Can you work these out from the drawing? Everything is in mm from the part's minimum corner. Coordinates: 2 decimals unless noted, no trailing zeros. Write each loop counter-clockwise with the first axis right and the second up, starting at its lowest first coordinate (ties: lowest second). Pieces come first, ordered by that corner, then holes.
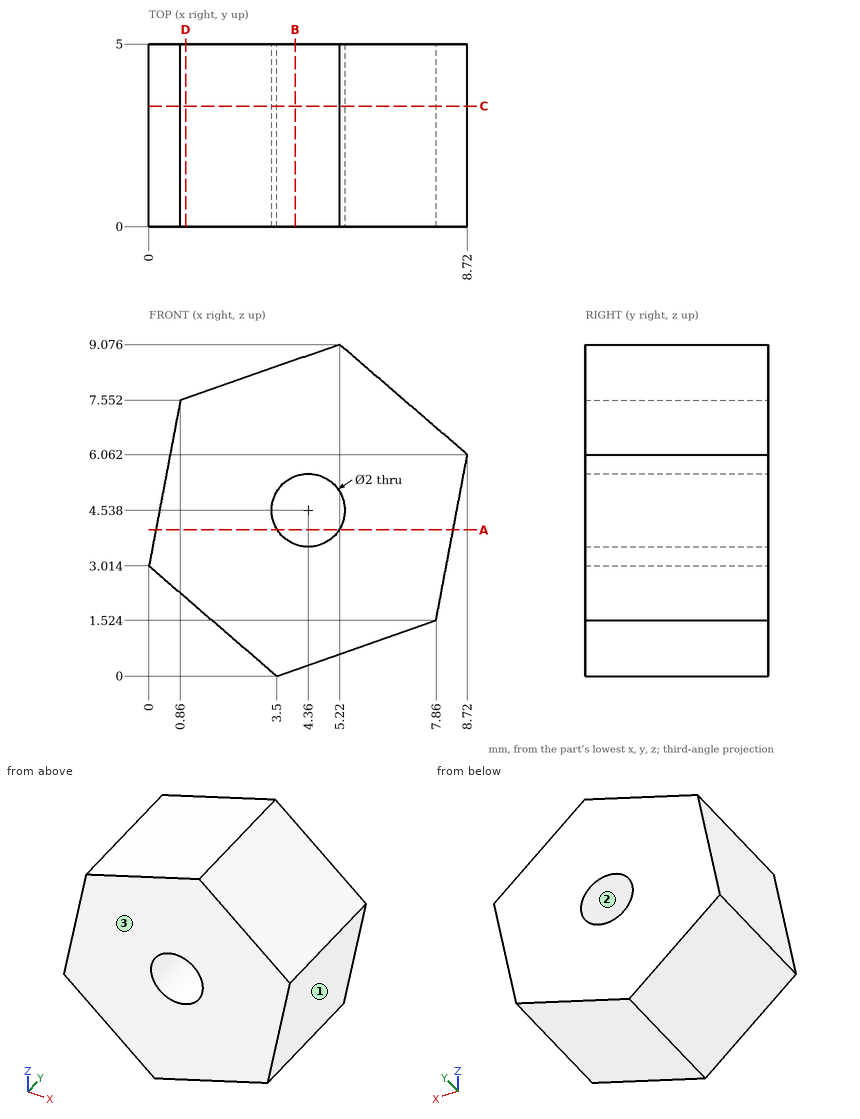
1. For pin 1 Ø3 at (y, z) = (3, 7) entering from -X, with a flat end and sliding along its axis, tell me the tip position at first contact or that it passes through.
2. Thinking about a two-plate mould opening in X: for the marked faces 1, 2 and 3, which applies, pulls with the +X half, pulls with the -X half, needs draft (parallel to the pull), parting line crosses it, or undercut?
3. I want a section at C-C (y = 3.3). List the corners of the cut face in (x, z) for me, then the cut area to 3 significant figures.
4. I want a section at D-D (x = 1). List the corners of the cut face in (y, z) for me.
5. If I drill on line 1 (Z direction, x = 4.75, y = 2.5); line 2 (Z direction, x = 4.25, y = 4.25); line 3 (X direction, y = 1.75, z = 4.5), over which ranges is the centre line in solid material (lowest first)?
6. I want a section at B-B (x = 4). List the corners of the cut face in (y, z) for me (1 decimal).
7. I want a section at A-A (z = 4). List the corners of the cut face in (x, y) for me.
Response values:
1. pin 1: stops at x = 0.47
2. face 1: pulls with the +X half
2. face 2: undercut
2. face 3: needs draft
3. outline: (0, 3.01) - (3.5, 0) - (7.86, 1.52) - (8.72, 6.06) - (5.22, 9.08) - (0.86, 7.55) - close; hole circle Ø2 at (4.36, 4.54)
3. area: 52.3 mm2
4. outline: (0, 2.15) - (5, 2.15) - (5, 7.6) - (0, 7.6) - close
5. line 1: z = 0.44 to 3.62, 5.46 to 8.91
5. line 2: z = 0.26 to 3.54, 5.53 to 8.74
5. line 3: x = 0.28 to 3.36, 5.36 to 8.42
6. outline: (0, 0.2) - (5, 0.2) - (5, 3.6) - (0, 3.6) - close; (0, 5.5) - (5, 5.5) - (5, 8.6) - (0, 8.6) - close
7. outline: (0.19, 0) - (3.52, 0) - (3.52, 5) - (0.19, 5) - close; (5.2, 0) - (8.33, 0) - (8.33, 5) - (5.2, 5) - close
